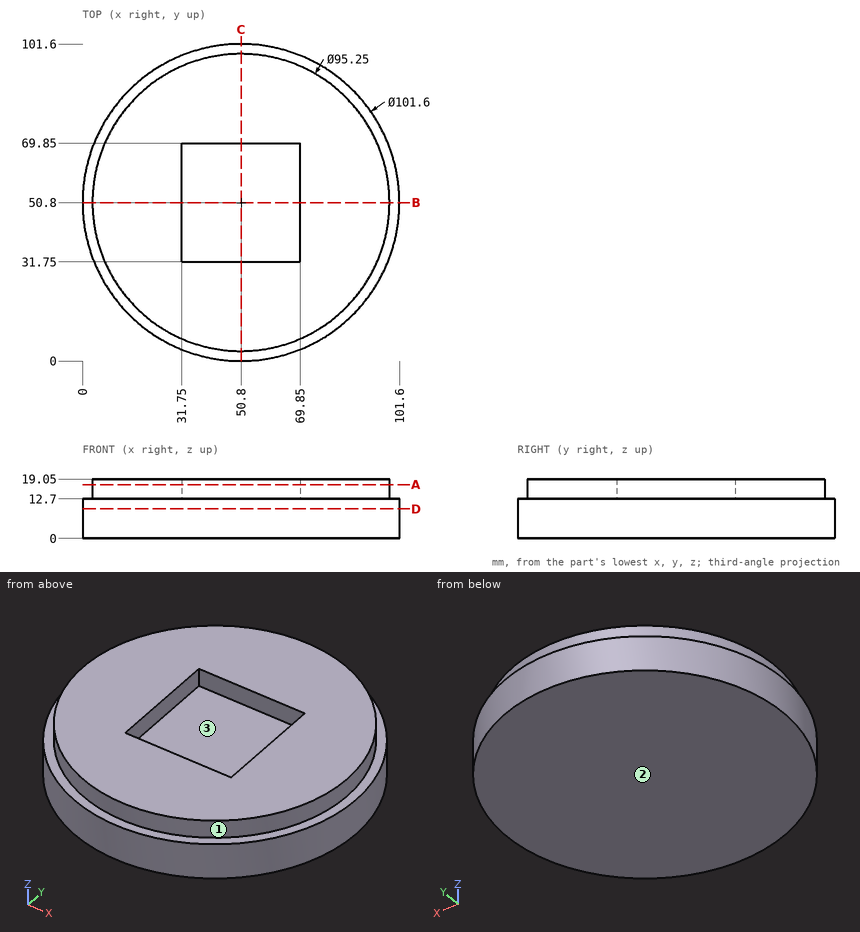
Can you work these out from the drawing? Everything is in mm from the part's minimum corner. Coordinates: 2 decimals unless noted, no trailing zeros. Write each loop counter-clockwise with the first axis right and the second up, starting at its lowest first coordinate (ties: lowest second). Pieces come first, ordered by that corner, then holes. Notation, with made-up numbers: (1.25, -24) - (11.25, -24) arc R16 ccw to (11.25, -6) - close; hole circle Ø7 at (34.5, 32.25). An arc over 180 degrees is marked (long way). Use a Markdown table: item, result.
Q1. Imagine slicing it at A-A (z = 17.25). List the corners of the cut face in (x, y) for me (3 decimals), and give its area (3 significant figures).
Geometry check:
| item | result |
|---|---|
| outline | circle Ø95.25 at (50.8, 50.8); hole (31.75, 31.75) - (69.85, 31.75) - (69.85, 69.85) - (31.75, 69.85) - close |
| area | 5,670 mm2 |
Q2. Please list where these lines run through material, in increasing order: L1, parallel to X at y = 50, z = 1; L2, parallel to X at y = 33.5, z = 14.25; L3, parallel to X at y = 58, z = 16.5.
Geometry check:
| item | result |
|---|---|
| L1 | x = 0.01 to 101.59 |
| L2 | x = 6.43 to 31.75, 69.85 to 95.17 |
| L3 | x = 3.72 to 31.75, 69.85 to 97.88 |
Q3. I'm going to push flat-ended pins straight in: pin 1 Ø19 at (x, y) = (47.5, 52.5) entering from +Z; pin 2 Ø1.9 at (x, z) = (53, 15.5) entering from -Y; pin 3 Ø1.5 at (x, y) = (87.5, 31) entering from -Z; pin 4 Ø6 at (x, z) = (43.5, 2) entering from -Y. Where does each tip first touch, or does it pass through?
Geometry check:
| item | result |
|---|---|
| pin 1 | stops at z = 12.7 |
| pin 2 | stops at y = 3.19 |
| pin 3 | stops at z = 0 |
| pin 4 | stops at y = 0.18 |
Q4. Imagine slicing it at B-B (y = 50.8). List the corners of the cut face in (x, z) for me (3 decimals), and give its area (3 significant figures).
Geometry check:
| item | result |
|---|---|
| outline | (0, 0) - (101.6, 0) - (101.6, 12.7) - (98.425, 12.7) - (98.425, 19.05) - (69.85, 19.05) - (69.85, 12.7) - (31.75, 12.7) - (31.75, 19.05) - (3.175, 19.05) - (3.175, 12.7) - (0, 12.7) - close |
| area | 1,650 mm2 |
Q5. Thinking about a two-plate mould opening in Y: for the marked faces 1, 2 and 3, which applies, +Y half, -Y half, draft (parallel to the pull), parting line (faces both ways), or undercut?
Geometry check:
| item | result |
|---|---|
| face 1 | parting line |
| face 2 | draft |
| face 3 | undercut |
Q6. Imagine slicing it at D-D (z = 9.5). List the corners of the cut face in (x, y) for me.
Geometry check:
| item | result |
|---|---|
| outline | circle Ø101.6 at (50.8, 50.8) |
